Verification items for this drawing (mm, ordinates from the low corner). A direction names the side the tool comes from. Coordinates: 2 decimals unless noted, no trailing zeros. Order: outer loops, then holes, each group sorted by start corner. A loop starts at its lowest first (then second) coordinate and runs counter-clockwise, first axis right, second up. Notation, with made-up numbers: (36.25, -18.75) - (79.25, -18.75) arc R26 ccw to (79.25, 17.25) - close; hole circle Ø7 at (78, 27.25). An arc over 180 degrees is marked (long way). One line per question, with ' | ' between items. Start each with the question number.
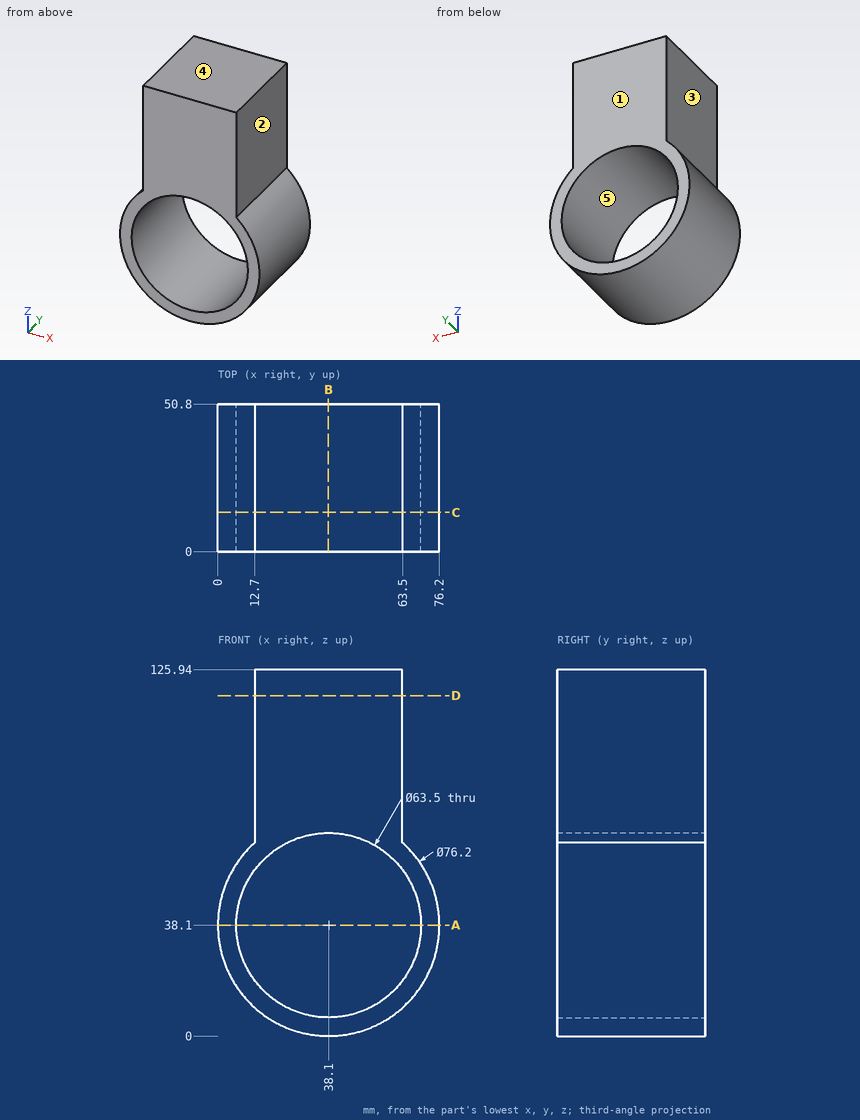
Item 1: Thickness scan on probe 1 along Z at (x, y) = (38, 39); probe 2 along X at (y, z) = (13.5, 38.1); probe 3 along X at (y, z) = (47, 111). Record the ranges inside material, lowest first. Write a range as from..to.
Item 2: Section check B-B (x = 38). Record the cut outline in (y, z).
Item 3: Set-up check for the marked faces 1 and 2: record each of +Z, -Z, +X, -X, +Y, -Y from which the full face is reachable in a straight line by a thin tool's end or side.
Item 4: Section check D-D (z = 117). Record the cut outline in (x, y).
Item 5: Section check A-A (z = 38.1). Record the cut outline in (x, y).
Item 6: Gauge pin test, flat ends, axial feed: pin 1 (1.5 mm diameter, centred on x = 67, y = 30.5, fed in from +Z) (1 decimal); pin 2 (2 mm diameter, centred on y = 34.5, z = 78, fed in from -X); pin 3 (8 mm diameter, centred on y = 20, z = 30.5, fed in from -X). Record the tip position at first contact, or that the pin passes through.
Item 7: Mould release check, pull along Z, two halves, no side actions. Record for the marked faces 3, 4 and 5: +Z half, -Z half, draft (parallel to the pull), parting line (faces both ways), or undercut.
Item 8: Section check C-C (y = 13.5). Record the cut outline in (x, z), then the cut area to 4 significant figures.
Completed:
1) probe 1: z = 0..6.35, 69.85..125.94 | probe 2: x = 0..6.35, 69.85..76.2 | probe 3: x = 12.7..63.5
2) outline: (0, 0) - (50.8, 0) - (50.8, 6.35) - (0, 6.35) - close; (0, 69.85) - (50.8, 69.85) - (50.8, 125.94) - (0, 125.94) - close
3) face 1: +Z, -Z, +X, -X, +Y | face 2: +Z, +X, +Y, -Y
4) outline: (12.7, 0) - (63.5, 0) - (63.5, 50.8) - (12.7, 50.8) - close
5) outline: (0, 0) - (6.35, 0) - (6.35, 50.8) - (0, 50.8) - close; (69.85, 0) - (76.2, 0) - (76.2, 50.8) - (69.85, 50.8) - close
6) pin 1: stops at z = 63.8 | pin 2: stops at x = 12.7 | pin 3: stops at x = 0.17
7) face 3: draft | face 4: +Z half | face 5: undercut
8) outline: (12.7, 66.5) arc R38.1 ccw (long way) to (63.5, 66.5) - (63.5, 125.94) - (12.7, 125.94) - close; hole circle Ø63.5 at (38.1, 38.1) | area: 4,075 mm^2
